from build123d import *

# Parameters (mm, degrees)
RESSALTO_EXTRUS_O1_DEPTH = 187
ESBO_O6_R                = 2.15
CORTE_EXTRUS_O1_DEPTH    = 101.765371804
ESBO_O8_R                = 4.15
CORTE_EXTRUS_O2_DEPTH    = 75


with BuildPart() as part:
    # Esboço1 → Ressalto-extrusão1 (new body)
    with BuildSketch(Plane.XY):
        Polygon((0, 0), (0, 27), (-100.765371804, 0), align=None)
    extrude(amount=RESSALTO_EXTRUS_O1_DEPTH)

    # Esboço6 → Corte-extrusão1 (cut, through all)
    with BuildSketch(Plane(origin=(0, 0, 0), x_dir=(0, 0, -1), z_dir=(1, 0, 0))):
        with Locations((-30, 13.5)):
            Circle(ESBO_O6_R)
        with Locations((-157, 13.5)):
            Circle(ESBO_O6_R)
    extrude(amount=-CORTE_EXTRUS_O1_DEPTH, mode=Mode.SUBTRACT)

    # Esboço8 → Corte-extrusão2 (cut)
    with BuildSketch(Plane(origin=(-100, 0, 0), x_dir=(0, 0, -1), z_dir=(1, 0, 0))):
        with Locations((-30, 13.5)):
            Circle(ESBO_O8_R)
        with Locations((-157, 13.5)):
            Circle(ESBO_O8_R)
    extrude(amount=CORTE_EXTRUS_O2_DEPTH, mode=Mode.SUBTRACT)


solid = part.part
Read the model definition and answer for the solid it produces. Units are mm, in the model's axes. A direction names the side the tool comes from. Coordinates: 2 decimals unless noted, no trailing zeros. Order: outer loops, then holes, each group sorted by start corner. A loop starts at its lowest first (then second) coordinate and runs counter-clockwise, first axis right, second up. Notation, with made-up numbers: (-24, 71) - (-18, 71) arc R19 cw to (-18, 106) - close; hole circle Ø6 at (87, 14). An arc over 180 degrees is marked (long way). Use one line per item in the form item = value.
(1) Straight lines are drawn through the part: L1, parallel to Z at x = -41, y = 13.5; L2, parallel to Z at x = -33, y = 12.5; L3, parallel to Y at x = -50, z = 157. For each, find the intervals that lie inside material, in ascending order.
Computed values:
L1 = 0 to 25.85, 34.15 to 152.85, 161.15 to 187
L2 = 0 to 25.97, 34.03 to 152.97, 161.03 to 187
L3 = 0 to 9.35
(2) Given pin 1 Ø4 at (y, z) = (13.5, 30) entering from -X; pin 2 Ø5 at (x, z) = (-36, 149.5) entering from +Y; pin 3 Ø5 at (y, z) = (16.5, 114.5) entering from +X; pin 4 Ø1.5 at (x, z) = (-31, 29) entering from +Y, each flat-ended and moving along its own axis, determine where each tip first touches the part or whether it passes through.
Computed values:
pin_1 = through
pin_2 = 18.02
pin_3 = 0
pin_4 = 18.89
(3) Section A-A, the plane y = 13.5 is taken. Give the vertices of the cut face in (x, z), then the cut area to 3 significant figures.
Computed values:
outline = (-50.38, 0) - (0, 0) - (0, 27.85) - (-25, 27.85) - (-25, 25.85) - (-50.38, 25.85) - close; (-50.38, 34.15) - (-25, 34.15) - (-25, 32.15) - (0, 32.15) - (0, 154.85) - (-25, 154.85) - (-25, 152.85) - (-50.38, 152.85) - close; (-50.38, 161.15) - (-25, 161.15) - (-25, 159.15) - (0, 159.15) - (0, 187) - (-50.38, 187) - close
area = 8,790 mm²
(4) Section B-B, the plane z = 157 is taken. Give the vertices of the cut face in (x, y).
Computed values:
outline = (-100.77, 0) - (0, 0) - (0, 11.35) - (-25, 11.35) - (-25, 9.35) - (-65.87, 9.35) - close; (-34.89, 17.65) - (-25, 17.65) - (-25, 15.65) - (0, 15.65) - (0, 27) - close
(5) Section C-C, the plane x = -12 is taken. Give the vertices of the cut face in (y, z).
Computed values:
outline = (0, 0) - (23.78, 0) - (23.78, 187) - (0, 187) - close; hole circle Ø4.3 at (13.5, 30); hole circle Ø4.3 at (13.5, 157)
(6) Section D-D, the plane x = -63 is taken. Give the vertices of the cut face in (y, z), then the cut area to 3 significant figures.
Computed values:
outline = (0, 0) - (10.12, 0) - (10.12, 27.59) arc R4.15 cw to (10.12, 32.41) - (10.12, 154.59) arc R4.15 cw to (10.12, 159.41) - (10.12, 187) - (0, 187) - close
area = 1,890 mm²
(7) Which of the six approach directions +Z, -Z, +X, -X, +Y, -Y give full straight-line access (tool end or side, diameter ignored) to faces 1 (the face through (-25, 12, 155)), 2 (the face through (0, 13, 92))?
Computed values:
face_1 = -X
face_2 = +Z, -Z, +X, +Y, -Y
(8) For a pull along Y with two mould halves and no side action, classify faces 3 (the face through (-49.68, 13.69, 92.19)), 4 (the face through (-12.32, 11.59, 29.01)), 5 (the face through (-25, 12, 28)), 6 (the face through (-29, 8, 187)) as pulls with the +Y half, pulls with the -Y half, needs draft (parallel to the pull), parting line crosses it, or undercut.
Computed values:
face_3 = pulls with the +Y half
face_4 = undercut
face_5 = undercut
face_6 = needs draft
